Geometry check sheet. Reference: the model listing, model coordinates, mm. A direction names the side the tool comes from. Round coordinates to 2 decimals unless told otherwise and drop trailing zeros. Order: outer loops, then holes, each group sorted by start corner. A loop starts at its lowest first (then second) coordinate and runs counter-clockwise, first axis right, second up.
(1) Cross-section at B-B on z = -1.8. Enter the section's corners in (x, y).
(2) Set-up check for faces 1 (the face through (12.878, 0, 2.5)), 2 (the face through (13.7, 1, -7)), 3 (the face through (12.878, 0, -2)), 4 (the face through (9, 0, -5.6)): record each of +Z, -Z, +X, -X, +Y, -Y from which the full face is reachable in a straight line by a thin tool's end or side.
(3) Gauge pin test, flat ends, axial feed: P1, Ø3, axis at x = 6, y = -1.5, coming from the -Z side; P2, Ø4.5, axis at x = 10, y = -0.5, coming from the +Z side; P3, Ø2, axis at x = 31.5, y = 1, coming from the -Z side. Record the tip position at first contact, or that the pin passes through.
(4) Cross-section at C-C on x = 56.5. Enter the section's corners in (y, z), and give its area (3 significant figures).
(5) Draft check along Z on faces 5 (the face through (9, 0, 2)), 6 (the face through (8.226, 0.481, -4.637)), 7 (the face through (11, -4, 1.2)), 8 (the face through (9, 0, 0.1)). Enter one of: pulls with the +Z half, pulls with the -Z half, needs draft (parallel to the pull), parting line crosses it, or undercut.
(6) Thickness scan on L1, parallel to Z at x = 8, y = 3.25; L2, parallel to X at y = 2.25, z = -3; L3, parallel to Y at x = 55, z = -4.75. Record the ranges inside material, lowest first.
(7) Cross-section at A-A on y = 0. Count the separate pieces of the cut face and the enclosed holes in it, and give its area (3 significant figures).
from build123d import *

# Parameters (mm, degrees)
SKETCH_3_W          = 10.261040874
SKETCH_3_H          = 1.404819466
CUT_EXTRUDE_1_DEPTH = 50
SKETCH_4_W          = 11.206560307
SKETCH_4_H          = 3.8
CUT_EXTRUDE_2_DEPTH = 50
SKETCH_7_R          = 1.6
CUT_EXTRUDE_4_DEPTH = 62.286866456


with BuildPart() as part:
    # 草图2 → 旋转1 (revolve)
    with BuildSketch(Plane.XY.offset(-1.8)):
        with BuildLine():
            Line((6.7, 5), (13.7, 5))
            Line((13.7, 5), (13.7, 6))
            Line((13.7, 6), (15.7, 6))
            Line((15.7, 6), (15.7, 3.35))
            Line((15.7, 3.35), (59.7, 3.35))
            Line((59.7, 3.35), (60.2, 2.85))
            Line((60.2, 2.85), (60.2, 0))
            Line((60.2, 0), (1.7, 0))
            ThreePointArc((1.7, 0), (3.164466094, 3.535533906), (6.7, 5))
        make_face()
    revolve(axis=Axis((60.2, 0, -1.8), (-1, 0, 0)))

    # 草图3 → 切除-拉伸1 (cut, symmetric)
    with BuildSketch(Plane(origin=(0, 0, -1.8), x_dir=(1, 0, 0), z_dir=(0, 1, 0))):
        with Locations((7.747323823, -4.502409733)):
            Rectangle(SKETCH_3_W, SKETCH_3_H)
        with Locations((7.747323823, 4.502409733)):
            Rectangle(SKETCH_3_W, SKETCH_3_H)
    extrude(amount=CUT_EXTRUDE_1_DEPTH, both=True, mode=Mode.SUBTRACT)

    # 草图4 → 切除-拉伸2 (cut, symmetric)
    with BuildSketch(Plane(origin=(0, 0, 0), x_dir=(1, 0, 0), z_dir=(0, 1, 0))):
        with Locations((7.274564107, 1.8)):
            Rectangle(SKETCH_4_W, SKETCH_4_H)
    extrude(amount=CUT_EXTRUDE_2_DEPTH, both=True, mode=Mode.SUBTRACT)

    # 草图7 → 切除-拉伸4 (cut, through all)
    with BuildSketch(Plane.XY.offset(2)):
        with Locations((6.7, 0)):
            Circle(SKETCH_7_R)
    extrude(amount=-CUT_EXTRUDE_4_DEPTH, mode=Mode.SUBTRACT)


solid = part.part
Found:
1. outline: (12.88, -5) - (13.7, -5) - (13.7, -6) - (15.7, -6) - (15.7, -3.35) - (59.7, -3.35) - (60.2, -2.85) - (60.2, 2.85) - (59.7, 3.35) - (15.7, 3.35) - (15.7, 6) - (13.7, 6) - (13.7, 5) - (12.88, 5) - close
2. face 1: +Z, -X, +Y, -Y
2. face 2: -X
2. face 3: -X, +Y, -Y
2. face 4: -Z, -X, +Y, -Y
3. P1: stops at z = -5.6
3. P2: stops at z = 2
3. P3: stops at z = -5.15
4. outline: circle Ø6.7 at (0, -1.8)
4. area: 35.3 mm2
5. face 5: pulls with the +Z half
5. face 6: needs draft
5. face 7: parting line crosses it
5. face 8: undercut
6. L1: z = -5.6 to -3.7, 0.1 to 2
6. L2: x = 12.88 to 60.2
6. L3: y = -1.59 to 1.59
7. separate pieces: 3
7. enclosed holes: 0
7. area: 357 mm2
